from build123d import *

# Parameters (mm, degrees)
F0_W            = 200
F0_H            = 213
F1_DEPTH        = 25
F3_DEPTH        = 70
F5_R            = 35.5
F6_DEPTH        = 130
F8_R            = 38.333334
F9_DEPTH        = 130
F10_R           = 20.5
F11_DEPTH       = 216.501
F12_R           = 20.5
F13_DEPTH       = 223.001
F14_W           = 60
F14_H           = 60
F15_DEPTH       = 10
F17_D           = 15
F17_CBORE_D     = 30
F17_CBORE_DEPTH = 10
F18_R           = 10
F19_R           = 15
F21_DEPTH       = 20
F22_R           = 10
F23_SIZE2       = 2
F23_SIZE        = 2


with BuildPart() as f1:
    # F0 (on Top) → F1 (new body)
    with BuildSketch(Plane.XY):
        Rectangle(F0_W, F0_H)
    extrude(amount=F1_DEPTH)

    # F2 (on face) → F3 (join)
    with BuildSketch(Plane.XY.offset(25)):
        with BuildLine():
            Line((-70, -26.5), (-70, -106.5))
            Line((-70, -106.5), (-55, -106.5))
            Line((-55, -106.5), (-55, -36.999305))
            ThreePointArc((-55, -36.999305), (4.246212, -10.746212), (30.499305, 48.5))
            Line((30.499305, 48.5), (100, 48.5))
            Line((100, 48.5), (100, 63.5))
            Line((100, 63.5), (20, 63.5))
            ThreePointArc((20, 63.5), (-6.36039, -0.13961), (-70, -26.5))
        make_face()
    extrude(amount=F3_DEPTH)

    # F5 (on offset) → F6 (join)
    with BuildSketch(Plane.XZ.offset(116.5)):
        with Locations((-62.5, 95)):
            Circle(F5_R)
    extrude(amount=-F6_DEPTH)

    # F8 (on offset) → F9 (join)
    with BuildSketch(Plane.YZ.offset(116.5)):
        with Locations((56.5, 95)):
            Circle(F8_R)
    extrude(amount=-F9_DEPTH)

    # F10 (on face) → F11 (cut, through all)
    with BuildSketch(Plane.YZ.offset(116.5)):
        with Locations((56.5, 95)):
            Circle(F10_R)
    extrude(amount=-F11_DEPTH, mode=Mode.SUBTRACT)

    # F12 (on face) → F13 (cut, through all)
    with BuildSketch(Plane.XZ.offset(116.5)):
        with Locations((-62.5, 95)):
            Circle(F12_R)
    extrude(amount=-F13_DEPTH, mode=Mode.SUBTRACT)

    # F14 (on face) → F15 (join)
    with BuildSketch(Plane.XY.offset(25)):
        with Locations((70, -76.5)):
            Rectangle(F14_W, F14_H)
    extrude(amount=F15_DEPTH)

    # F17 (through all)
    with Locations(Plane.XY.offset(35)):
        with Locations((70, -76.5)):
            CounterBoreHole(F17_D / 2, F17_CBORE_D / 2, F17_CBORE_DEPTH)

    # F18
    f18_edges = [f1.edges().sort_by_distance(p)[0] for p in [
        (100, 106.5, 12.5),
        (100, -106.5, 17.5),
        (-100, -106.5, 12.5),
        (-100, 106.5, 12.5),
    ]]
    fillet(f18_edges, radius=F18_R)

    # F19
    f19_edges = [f1.edges().sort_by_distance(p)[0] for p in [
        (40, -46.5, 30),
    ]]
    fillet(f19_edges, radius=F19_R)

    # F20 (on face) → F21 (cut)
    with BuildSketch(Plane.XY.offset(25)):
        with BuildLine():
            Line((-46, -43.195626), (-46, -97.5))
            Line((-46, -97.5), (31, -97.5))
            Line((31, -97.5), (31, -62.762026))
            ThreePointArc((31, -62.762026), (38.005991, -44.505991), (56.262026, -37.5))
            Line((56.262026, -37.5), (91, -37.5))
            Line((91, -37.5), (91, 39.5))
            Line((91, 39.5), (36.695626, 39.5))
            ThreePointArc((36.695626, 39.5), (10.610173, -17.110173), (-46, -43.195626))
        make_face()
    extrude(amount=-F21_DEPTH, mode=Mode.SUBTRACT)

    # F22
    f22_edges = [f1.edges().sort_by_distance(p)[0] for p in [
        (36.695626, 39.5, 15),
        (-46, -43.195626, 15),
        (91, 39.5, 15),
        (91, -37.5, 15),
        (31, -97.5, 15),
        (-46, -97.5, 15),
    ]]
    fillet(f22_edges, radius=F22_R)

    # F23
    f23_edges = [f1.edges().sort_by_distance(p)[0] for p in [
        (-83, -116.5, 95),
        (116.5, 36, 95),
        (-13.5, 36, 95),
        (-83, 13.5, 95),
    ]]
    chamfer(f23_edges, length=F23_SIZE, length2=F23_SIZE2)


solid = f1.part
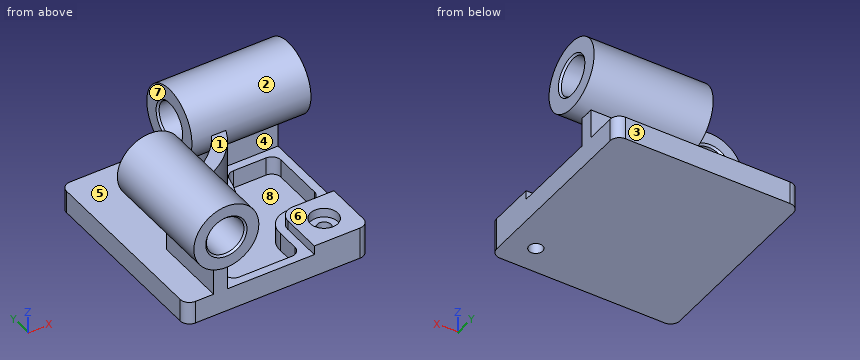
Verification items for the finished model (mm, model axes). Face numbers are marked on the shaded views. A direction names the side the tool comes from. Coordinates: 2 decimals unless noted, no trailing zeros. Order: outer loops, then holes, each group sorted by start corner. A loop starts at its lowest first (then second) coordinate and runs counter-clockwise, first axis right, second up.
1. Set-up check for the marked faces 5, 6, 7 and 8: record each of +Z, -Z, +X, -X, +Y, -Y from which the full face is reachable in a straight line by a thin tool's end or side.
Results found:
face 5: -X, +Y
face 6: +Z, +X, -Y
face 7: +Z, -X, +Y
face 8: none
2. Sectioned sample at B-B, the plane y = -76.5. Record the cut outline in (x, z).
Results found:
outline: (-100, 0) - (62.5, 0) - (62.5, 25) - (55, 25) - (55, 35) - (40, 35) - (40, 25) - (31, 25) - (31, 5) - (-46, 5) - (-46, 25) - (-55, 25) - (-55, 60.3) arc R35.5 ccw (long way) to (-70, 60.3) - (-70, 25) - (-100, 25) - close; (77.5, 0) - (100, 0) - (100, 35) - (85, 35) - (85, 25) - (77.5, 25) - close; hole circle Ø41 at (-62.5, 95)
3. Scan lines: line 1 (X direction, y = -76, z = 31); line 2 (Y direction, x = 70, z = 29); line 3 (Y direction, x = 70, z = 9.5). Record each from-to range of solid material in increasing order.
Results found:
line 1: x = -70 to -55, 40 to 55.01, 84.99 to 100
line 2: y = -106.5 to -91.5, -61.5 to -46.5, 48.5 to 63.5
line 3: y = -106.5 to -84, -69 to -37.5, 39.5 to 106.5
4. Sectioned sample at D-D, the plane x = -62.5. Record the cut outline in (y, z).
Results found:
outline: (-116.5, 59.5) - (-106.5, 59.5) - (-106.5, 0) - (106.5, 0) - (106.5, 25) - (-26.19, 25) - (-26.19, 59.5) - (13.5, 59.5) - (13.5, 72.5) - (11.5, 74.5) - (-114.5, 74.5) - (-116.5, 72.5) - close; (-116.5, 117.5) - (-114.5, 115.5) - (11.5, 115.5) - (13.5, 117.5) - (13.5, 130.5) - (-116.5, 130.5) - close
5. Release check for a two-part mould opening along Z. For the marked faces 1, 2, 3 and 4 record: +Z half, -Z half, draft (parallel to the pull), parting line (faces both ways), or undercut.
Results found:
face 1: +Z half
face 2: undercut
face 3: draft
face 4: undercut
6. Sectioned sample at A-A, the plane z = 32. Record the cut outline in (x, y), and give its area (3 significant figures).
Results found:
outline: (-70, -106.5) - (-55, -106.5) - (-55, -37) arc R90 ccw to (30.5, 48.5) - (100, 48.5) - (100, 63.5) - (20, 63.5) arc R90 cw to (-70, -26.5) - close; (40, -106.5) - (90, -106.5) arc R10 ccw to (100, -96.5) - (100, -46.5) - (55, -46.5) arc R15 ccw to (40, -61.5) - close; hole circle Ø30 at (70, -76.5)
area: 6,930 mm2
7. Go/stop test with flat-tipped pins: pin 1 Ø1 at (x, z) = (9.5, 69) entering from -Y; pin 2 Ø4 at (x, y) = (-37, -48) entering from +Z; pin 3 Ø10.5 at (y, z) = (-56.5, 34.5) entering from +X. Record where each tip stops, or that it passes through.
Results found:
pin 1: stops at y = -5.61
pin 2: stops at z = 121.61
pin 3: stops at x = 100
8. Sectioned sample at C-C, the plane y = 56.5. Record the cut outline in (x, z).
Results found:
outline: (-100, 0) - (100, 0) - (100, 56.67) - (116.5, 56.67) - (116.5, 72.5) - (114.5, 74.5) - (-11.5, 74.5) - (-13.5, 72.5) - (-13.5, 56.67) - (19.73, 56.67) - (19.73, 25) - (-100, 25) - close; (-13.5, 117.5) - (-11.5, 115.5) - (114.5, 115.5) - (116.5, 117.5) - (116.5, 133.33) - (-13.5, 133.33) - close
